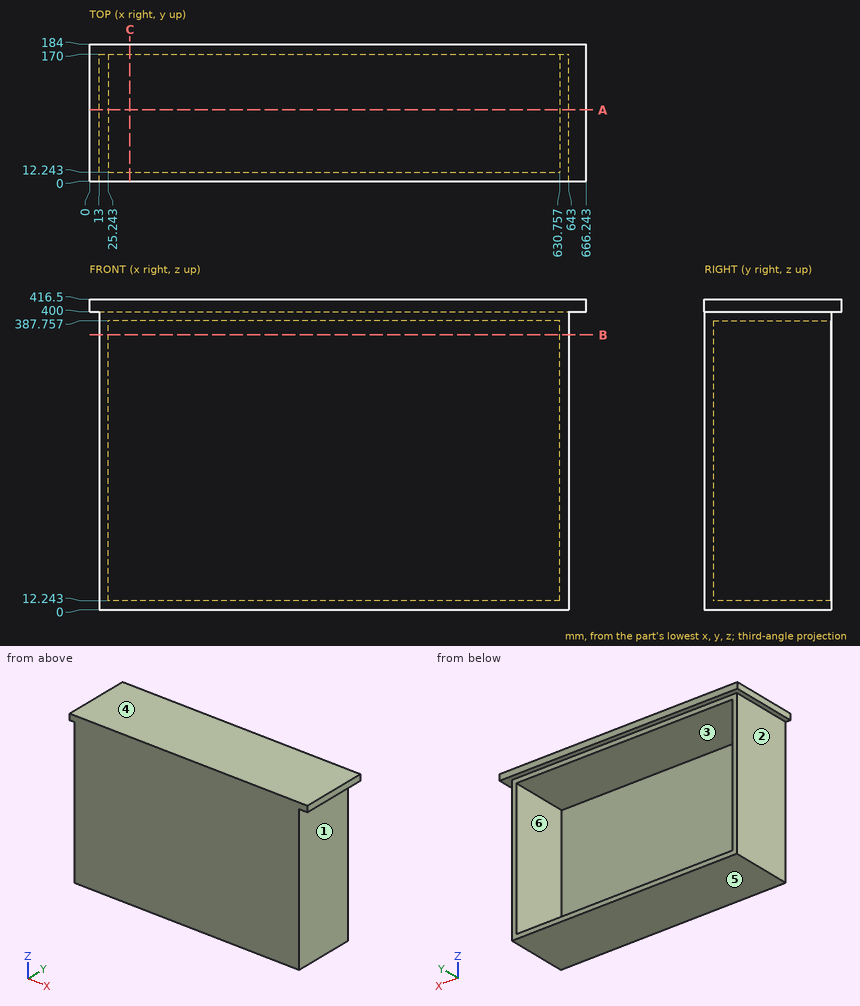
Print and shaded views of the part. All mm, measured from the part's lowest x, y and z. A direction names the side the tool comes from. Round coordinates to 2 decimals unless told otherwise and drop trailing zeros. Write each loop counter-clockwise with the first axis right and the second up, starting at its lowest first coordinate (ties: lowest second). Pieces come first, ordered by that corner, then holes. Notation, with made-up numbers: (24, -31.5) -> (63, -31.5) arc R19 ccw to (63, 4.5) -> close; hole circle Ø5 at (-40, 25). An arc over 180 degrees is marked (long way). Return JSON: item names as keys, results as strings. Group by question number.
Q1. Saw through at C-C on x = 54. Write the cut outline in (y, z).
Q2. Saw through at B-B on z = 368.5. Write the cut outline in (x, y), plus the area to 3 significant figures.
Q3. Mould opens along Z. For the marked faces 4, 5 and 6 say: pulls with the +Z half, pulls with the -Z half, needs draft (parallel to the pull), parting line crosses it, or undercut.
Q4. Pin check, flat tips, straight feed: pin 1 (12 mm diameter, centred on y = 149.5, z = 168.5, fed in from +X); pin 2 (1.5 mm diameter, centred on x = 548, z = 193.5, fed in from +Y); pin 3 (3 mm diameter, centred on y = 81.5, z = 226, fed in from -X). Stop position of each tip, or through.
Q5. Probe L1, parallel to X at y = 94, z = 327; L2, parallel to Z at x = 576.5, y = 68.5; L3, parallel to Y at x = 135.5, z = 137.5. List the from-to ranges inside material, lowest first. Write a range as [from, to].
Q6. Saw through at A-A on y = 95.5. Write the cut outline in (x, z), plus the area to 3 significant figures.
Q7. Which spindle directions (+Z, -Z, +X, -X, +Y, -Y) get a long thin tool onto all of the face, cutting with end or side? Do the marked faces 1, 2 and 3. Say none if no direction does.
Answer:
{
 "1": {"outline": "(0, 0) -> (170, 0) -> (170, 12.24) -> (12.24, 12.24) -> (12.24, 387.76) -> (170, 387.76) -> (170, 400) -> (184, 400) -> (184, 416.5) -> (0, 416.5) -> close"},
 "2": {"outline": "(13, 0) -> (643, 0) -> (643, 170) -> (630.76, 170) -> (630.76, 12.24) -> (25.24, 12.24) -> (25.24, 170) -> (13, 170) -> close", "area": "11,600 mm2"},
 "3": {"face 4": "pulls with the +Z half", "face 5": "pulls with the -Z half", "face 6": "undercut"},
 "4": {"pin 1": "x = 643", "pin 2": "y = 12.24", "pin 3": "x = 13"},
 "5": {"L1": "[13, 25.24], [630.76, 643]", "L2": "[0, 12.24], [387.76, 416.5]", "L3": "[0, 12.24]"},
 "6": {"outline": "(0, 400) -> (13, 400) -> (13, 0) -> (643, 0) -> (643, 400) -> (666.24, 400) -> (666.24, 416.5) -> (0, 416.5) -> close; hole (25.24, 12.24) -> (630.76, 12.24) -> (630.76, 387.76) -> (25.24, 387.76) -> close", "area": "35,600 mm2"},
 "7": {"face 1": "-Z, +X, +Y, -Y", "face 2": "-Z, -X, +Y, -Y", "face 3": "+Y"}
}
